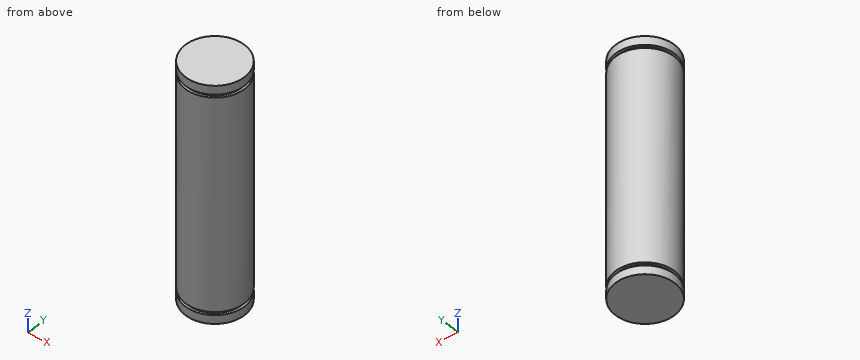
```python
from build123d import *

# Parameters (mm, degrees)
SKETCH_1_R          = 12.5
EXTRUDE_1_DEPTH     = 5
SKETCH_1_2_R        = 12.5
EXTRUDE_2_DEPTH     = 95
SKETCH_2_OUTSIDE_W  = 48.214
SKETCH_2_OUTSIDE_H  = 48.214
SKETCH_2_OUTSIDE_R  = 11.45
CUT_EXTRUDE_1_DEPTH = 1.3
SKETCH_3_OUTSIDE_W  = 48.214
SKETCH_3_OUTSIDE_H  = 48.214
SKETCH_3_OUTSIDE_R  = 11.45
CUT_EXTRUDE_2_DEPTH = 1.3


with BuildPart() as part:
    # 草图1 → 凸台-拉伸1 (new body)
    with BuildSketch(Plane.XY.offset(5503)):
        with Locations((1309.324811799, 736.635546363)):
            Circle(SKETCH_1_R)
    extrude(amount=EXTRUDE_1_DEPTH)

    # 草图1<2> → 凸台-拉伸2 (add)
    with BuildSketch(Plane.XY.offset(5503)):
        with Locations((1309.324811799, 736.635546363)):
            Circle(SKETCH_1_2_R)
    extrude(amount=-EXTRUDE_2_DEPTH)

    # 草图2 outside → 切除-拉伸1 (cut)
    with BuildSketch(Plane.XY.offset(5503)):
        with Locations((1309.325, 736.636)):
            Rectangle(SKETCH_2_OUTSIDE_W, SKETCH_2_OUTSIDE_H)
        with Locations((1309.324811799, 736.635546363)):
            Circle(SKETCH_2_OUTSIDE_R, mode=Mode.SUBTRACT)
    extrude(amount=CUT_EXTRUDE_1_DEPTH, mode=Mode.SUBTRACT)

    # 草图3 outside → 切除-拉伸2 (cut)
    with BuildSketch(Plane(origin=(0, 0, 5413), x_dir=(-1, 0, 0), z_dir=(0, 0, -1))):
        with Locations((-1309.325, 736.636)):
            Rectangle(SKETCH_3_OUTSIDE_W, SKETCH_3_OUTSIDE_H)
        with Locations((-1309.324811799, 736.635546363)):
            Circle(SKETCH_3_OUTSIDE_R, mode=Mode.SUBTRACT)
    extrude(amount=CUT_EXTRUDE_2_DEPTH, mode=Mode.SUBTRACT)


solid = part.part
```
CAD build for the part. Positions are in the model's coordinates, mm. Round coordinates to 2 decimals unless told otherwise and drop trailing zeros. Write each loop counter-clockwise with the first axis right and the second up, starting at its lowest first coordinate (ties: lowest second). Pieces come first, ordered by that corner, then holes. Notation, with made-up numbers: (-1.5, 57.25) -> (9.5, 57.25) arc R21 ccw to (9.5, 85.25) -> close; hole circle Ø11 at (25, 71). An arc over 180 degrees is marked (long way). Answer in a Markdown table with one row per item. Add a question column.
Item 1: Saw through at C-C, the plane z = 5452. Write the cut outline in (x, y).
Item 2: Drill centre lines: line 1 (Z direction, x = 1299, y = 742.75); line 2 (X direction, y = 731.75, z = 5447); line 3 (X direction, y = 726.5, z = 5452). Where is each one in solid material? Low to high. Write a range as from..to.
Item 3: Saw through at B-B, the plane y = 744. Write the cut outline in (x, z).
Item 4: Drop flat-ended pins along their axis: pin 1 Ø4 at (x, z) = (1313.5, 5426.5) entering from +Y; pin 2 Ø1.5 at (y, z) = (746.5, 5486) entering from -X; pin 3 Ø1.5 at (y, z) = (739, 5497) entering from -X; pin 4 Ø6 at (y, z) = (735.5, 5453) entering from -X. Give the stop position or say it passes through.
Item 5: Saw through at A-A, the plane x = 1299. Write the cut outline in (y, z), then the cut area to 3 significant figures.
Findings below:
| question | item | result |
|---|---|---|
| 1 | outline | circle Ø25 at (1309.32, 736.64) |
| 2 | line 1 | z = 5408..5411.7, 5413..5503, 5504.3..5508 |
| 2 | line 2 | x = 1297.82..1320.83 |
| 2 | line 3 | x = 1302.01..1316.64 |
| 3 | outline | (1299.22, 5408) -> (1319.43, 5408) -> (1319.43, 5411.7) -> (1318.09, 5411.7) -> (1318.09, 5413) -> (1319.43, 5413) -> (1319.43, 5503) -> (1318.09, 5503) -> (1318.09, 5504.3) -> (1319.43, 5504.3) -> (1319.43, 5508) -> (1299.22, 5508) -> (1299.22, 5504.3) -> (1300.56, 5504.3) -> (1300.56, 5503) -> (1299.22, 5503) -> (1299.22, 5413) -> (1300.56, 5413) -> (1300.56, 5411.7) -> (1299.22, 5411.7) -> close |
| 4 | pin 1 | stops at y = 748.94 |
| 4 | pin 2 | stops at x = 1300.77 |
| 4 | pin 3 | stops at x = 1296.93 |
| 4 | pin 4 | stops at x = 1296.82 |
| 5 | outline | (729.59, 5408) -> (743.68, 5408) -> (743.68, 5411.7) -> (741.59, 5411.7) -> (741.59, 5413) -> (743.68, 5413) -> (743.68, 5503) -> (741.59, 5503) -> (741.59, 5504.3) -> (743.68, 5504.3) -> (743.68, 5508) -> (729.59, 5508) -> (729.59, 5504.3) -> (731.69, 5504.3) -> (731.69, 5503) -> (729.59, 5503) -> (729.59, 5413) -> (731.69, 5413) -> (731.69, 5411.7) -> (729.59, 5411.7) -> close |
| 5 | area | 1,400 mm^2 |
